Design review of the part built by this model. Coordinates are the model's own, in mm. A direction names the side the tool comes from. Give positions to 0.01 mm unless a question says otherwise; leave off trailing zeros. Order: outer loops, then holes, each group sorted by start corner. A loop starts at its lowest first (then second) coordinate and runs counter-clockwise, first axis right, second up. Notation, with made-up numbers: (24, 28) -> (56, 28) arc R16 cw to (56, 50) -> close; hole circle Ø11 at (35, 68). An arc over 180 degrees is marked (long way). One line per item, written item: value. Start each with the question number.
1) Consider section C-C (z = 45). State the section outline as (x, y) points, plus the area to 3 significant figures.
2) Tool access review of faces 5 (the face through (-17, -55, 33.5)), 6 (the face through (83, 1, 15)), 7 (the face through (-1, 55, 25)), 8 (the face through (77.193, -41.467, 12.535)): name each direction out of +Z, -Z, +X, -X, +Y, -Y from which nothing blocks a thin tool from reaching the whole face with its end or side.
3) Consider section B-B (y = 2). State the section outline as (x, z) points, plus the area to 4 significant figures.
4) Consider section A-A (x = 43.5). State the section outline as (y, z) points.
5) Wall thickness on line 1 along Y through (x, z) = (75.5, 11.4) (3 decimals); line 2 along Z through (x, y) = (-9, -58); line 3 along Y through (x, z) = (-24, 10.5): over which ranges is each line inside the solid? List them lowest first. Write a range as from..to.
6) The part is to be moulded in two halves that separate along Y. For faces 1 (the face through (-20, -60, 36)), 2 (the face through (88.859, 58.797, 12.675)), 3 (the face through (-17, -55, 28.5)), 4 (the face through (-80.5, 0, 12)), say which applies: released by +Y, released by -Y, zero draft, split by the parting line, or undercut.
7) For pin 1 (2 mm diameter, centred on x = -7, y = -12.5, fed in from +Z); pin 2 (1.5 mm diameter, centred on y = -57, z = 31, fed in from +X); pin 3 (4.5 mm diameter, centred on x = -67, z = 90, fed in from -Y); pin 4 (5.5 mm diameter, centred on x = -67, z = 41, fed in from +Y), all flat-tipped, find the tip position at first contact; note any pin that passes through.
from build123d import *

# Parameters (mm, degrees)
SKETCH_W        = 161
SKETCH_H        = 101
PAD_DEPTH       = 10
SKETCH001_W     = 15
SKETCH001_H     = 15
PAD001_DEPTH    = 5
SKETCH003_R     = 1.775
HOLE_DEPTH      = 5
HOLE_TIPS_R     = 1.775
SKETCH005_W     = 180
SKETCH005_H     = 120
SKETCH005_W_2   = 161
SKETCH005_H_2   = 101
PAD002_DEPTH    = 25
SKETCH006_W     = 9.5
SKETCH006_H     = 101
POCKET_DEPTH    = 10
SKETCH007_W     = 9.5
SKETCH007_H     = 101
POCKET001_DEPTH = 10
SKETCH008_W     = 90
SKETCH008_H     = 9.5
PAD003_DEPTH    = 70
SKETCH009_R     = 1.75
HOLE001_DEPTH   = 25
SKETCH010_W     = 8
SKETCH010_H     = 5
POCKET002_DEPTH = 10
FILLET_R        = 1
FILLET001_R     = 4


with BuildPart() as part:
    # Sketch → Pad (new body)
    with BuildSketch(Plane.XY):
        Rectangle(SKETCH_W, SKETCH_H)
    extrude(amount=PAD_DEPTH)

    # Sketch001 (on Face6 of Pad) → Pad001 (join)
    with BuildSketch(Plane.XY.offset(10)):
        with Locations((-73, 43)):
            Rectangle(SKETCH001_W, SKETCH001_H)
        with Locations((-73, -43)):
            Rectangle(SKETCH001_W, SKETCH001_H)
        with Locations((73, -43)):
            Rectangle(SKETCH001_W, SKETCH001_H)
        with Locations((73, 43)):
            Rectangle(SKETCH001_W, SKETCH001_H)
    extrude(amount=PAD001_DEPTH)

    # Sketch003 (on Face25 of Pad001) → Hole (cut)
    with BuildSketch(Plane.XY.offset(15)):
        with Locations((-76.5, -46.5)):
            Circle(SKETCH003_R)
        with Locations((-76.5, 46.5)):
            Circle(SKETCH003_R)
        with Locations((75.5, -42)):
            Circle(SKETCH003_R)
        with Locations((75.5, 42)):
            Circle(SKETCH003_R)
    extrude(amount=-HOLE_DEPTH, mode=Mode.SUBTRACT)

    # Hole tips → Hole tip 1 section 0
    with BuildSketch(Plane.XY.offset(10), mode=Mode.PRIVATE) as hole_tip_1_s0:
        with Locations((-76.5, -46.5)):
            Circle(HOLE_TIPS_R)
    loft([hole_tip_1_s0.sketch, Vertex(-76.5, -46.5, 8.933472)], mode=Mode.SUBTRACT)

    # Hole tips → Hole tip 2 section 0
    with BuildSketch(Plane.XY.offset(10), mode=Mode.PRIVATE) as hole_tip_2_s0:
        with Locations((-76.5, 46.5)):
            Circle(HOLE_TIPS_R)
    loft([hole_tip_2_s0.sketch, Vertex(-76.5, 46.5, 8.933472)], mode=Mode.SUBTRACT)

    # Hole tips → Hole tip 3 section 0
    with BuildSketch(Plane.XY.offset(10), mode=Mode.PRIVATE) as hole_tip_3_s0:
        with Locations((75.5, -42)):
            Circle(HOLE_TIPS_R)
    loft([hole_tip_3_s0.sketch, Vertex(75.5, -42, 8.933472)], mode=Mode.SUBTRACT)

    # Hole tips → Hole tip 4 section 0
    with BuildSketch(Plane.XY.offset(10), mode=Mode.PRIVATE) as hole_tip_4_s0:
        with Locations((75.5, 42)):
            Circle(HOLE_TIPS_R)
    loft([hole_tip_4_s0.sketch, Vertex(75.5, 42, 8.933472)], mode=Mode.SUBTRACT)

    # Sketch005 → Pad002 (join)
    with BuildSketch(Plane.XY):
        Rectangle(SKETCH005_W, SKETCH005_H)
        Rectangle(SKETCH005_W_2, SKETCH005_H_2, mode=Mode.SUBTRACT)
    extrude(amount=PAD002_DEPTH)

    # Sketch006 (on Face7 of Pad002) → Pocket (cut)
    with BuildSketch(Plane.XY.offset(25)):
        with Locations((85.25, 0)):
            Rectangle(SKETCH006_W, SKETCH006_H)
    extrude(amount=-POCKET_DEPTH, mode=Mode.SUBTRACT)

    # Sketch007 (on Face7 of Pocket) → Pocket001 (cut)
    with BuildSketch(Plane.XY.offset(25)):
        with Locations((-85.25, 0)):
            Rectangle(SKETCH007_W, SKETCH007_H)
    extrude(amount=-POCKET001_DEPTH, mode=Mode.SUBTRACT)

    # Sketch008 (on Face7 of Pocket001) → Pad003 (join)
    with BuildSketch(Plane.XY.offset(25)):
        with Locations((-45, -55.25)):
            Rectangle(SKETCH008_W, SKETCH008_H)
    extrude(amount=PAD003_DEPTH)

    # Sketch009 (on Face18 of Pad003) → Hole001 (cut)
    with BuildSketch(Plane(origin=(0, -50.5, 0), x_dir=(-1, 0, 0), z_dir=(0, 1, 0))):
        with Locations((67, 90)):
            Circle(SKETCH009_R)
        with Locations((9, 90)):
            Circle(SKETCH009_R)
        with Locations((9, 41)):
            Circle(SKETCH009_R)
        with Locations((67, 41)):
            Circle(SKETCH009_R)
    extrude(amount=-HOLE001_DEPTH, mode=Mode.SUBTRACT)

    # Sketch010 (on Face18 of Hole001) → Pocket002 (cut)
    with BuildSketch(Plane(origin=(0, -50.5, 0), x_dir=(-1, 0, 0), z_dir=(0, 1, 0))):
        with Locations((16.7, 31)):
            Rectangle(SKETCH010_W, SKETCH010_H)
    extrude(amount=-POCKET002_DEPTH, mode=Mode.SUBTRACT)

    # Fillet
    fillet_edges = [part.edges().sort_by_distance(p)[0] for p in [
        (-20.7, -55.25, 33.5),
        (-12.7, -55.25, 33.5),
        (-20.7, -55.25, 28.5),
        (-12.7, -55.25, 28.5),
    ]]
    fillet(fillet_edges, radius=FILLET_R)

    # Fillet001
    fillet001_edges = [part.edges().sort_by_distance(p)[0] for p in [
        (90, -60, 12.5),
        (90, 60, 12.5),
        (-90, 60, 12.5),
        (-90, -60, 12.5),
        (-90, -60, 60),
    ]]
    fillet(fillet001_edges, radius=FILLET001_R)


solid = part.part
Checked values:
1. outline: (-90, -56) arc R4 ccw to (-86, -60) -> (0, -60) -> (0, -50.5) -> (-90, -50.5) -> close
1. area: 852 mm^2
2. face 5: +Y, -Y
2. face 6: +Z, +X, -X
2. face 7: +Z, +X, -X, +Y
2. face 8: +Z
3. outline: (-90, 0) -> (90, 0) -> (90, 15) -> (80.5, 15) -> (80.5, 10) -> (-80.5, 10) -> (-80.5, 15) -> (-90, 15) -> close
3. area: 1,895 mm^2
4. outline: (-60, 0) -> (60, 0) -> (60, 25) -> (50.5, 25) -> (50.5, 10) -> (-50.5, 10) -> (-50.5, 25) -> (-60, 25) -> close
5. line 1: y = -60..-43.775, -40.225..-35.5, 35.5..40.225, 43.775..60
5. line 2: z = 0..39.25, 42.75..88.25, 91.75..95
5. line 3: y = -60..-50.5, 50.5..60
6. face 1: released by -Y
6. face 2: released by +Y
6. face 3: zero draft
6. face 4: undercut
7. pin 1: stops at z = 10
7. pin 2: stops at x = 0
7. pin 3: stops at y = -60
7. pin 4: stops at y = -50.5
